Can you work these out from the model? Positions are in its coordinate system, mm. A direction names the side the tool comes from. Coordinates: 2 decimals unless noted, no trailing zeros. Order: outer loops, then holes, each group sorted by start corner. A loop starts at its lowest first (then second) coordinate and runs counter-clockwise, first axis right, second up. Notation, with made-up numbers: (43, 11) - (69, 11) arc R18 ccw to (69, 45) - close; hole circle Ø7 at (34, 83). An arc over 180 degrees is marked (long way). Return JSON: item names as keys, results as strings. Group by question number.
1) For pin 1 Ø3 at (x, z) = (-13.5, -8.5) entering from +Y; pin 2 Ø8.5 at (y, z) = (12.34, -11.91) entering from +X; pin 3 Ø4 at (y, z) = (16.5, -9) entering from -X, each with a flat end and sliding along its axis, tell me the tip position at first contact or that it passes through.
2) Which directions (+Z, -Z, +X, -X, +Y, -Y) give clear straight access to the entire face, cutting with the end or side of a thin tool? Please do faces 1 (the face through (0, 19, -12)), 2 (the face through (-3, 4, -23.81)).
3) Imagine slicing it at B-B (z = -12). Write out the boundary of the cut face in (x, y).
4) Imagine slicing it at A-A (y = 13.5). Write out the boundary of the cut face in (x, z), and give its area (3 significant figures).
5) Imagine slicing it at D-D (y = 16). Write out the boundary of the cut face in (x, z).
6) If we mould it in two halves opening along X, with no side actions, what happens to faces 3 (the face through (-6, 0, -12)), 4 (the face through (-16.026, 2, -12)), 5 (the face through (5, 7, -9))? For each: pulls with the +X half, pulls with the -X half, needs draft (parallel to the pull), parting line crosses it, or undercut.
7) If I drill on line 1 along Y through (x, z) = (-7.75, -14); line 2 along Y through (x, z) = (3, -22.25), over which ranges is the centre line in solid material (lowest first)?
```python
from build123d import *

# Parameters (mm, degrees)
SKETCH2_W           = 16.026033158
SKETCH2_H           = 23.810106406
BOSS_EXTRUDE1_DEPTH = 5
SKETCH3_R           = 5.388558838
BOSS_EXTRUDE2_DEPTH = 5


with BuildPart() as part:
    # Sketch2 → Boss-Extrude1 (new body)
    with BuildSketch(Plane(origin=(0, 0, 0), x_dir=(1, 0, 0), z_dir=(0, 1, 0))):
        with Locations((-8.013016579, 11.905053203)):
            Rectangle(SKETCH2_W, SKETCH2_H)
    extrude(amount=BOSS_EXTRUDE1_DEPTH)

    # Sketch3 → Boss-Extrude2 (add)
    with BuildSketch(Plane(origin=(0, 0, 0), x_dir=(0, 0, -1), z_dir=(1, 0, 0))):
        with BuildLine():
            Line((0, 0), (0, 12.341839421))
            ThreePointArc((0, 12.341839421), (11.905053203, 24.246892624), (23.810106406, 12.341839421))
            Line((23.810106406, 12.341839421), (23.810106406, 0))
            Line((23.810106406, 0), (0, 0))
        make_face()
        with Locations((11.905053203, 12.341839421)):
            Circle(SKETCH3_R, mode=Mode.SUBTRACT)
    extrude(amount=BOSS_EXTRUDE2_DEPTH)


solid = part.part
```
Calculated:
{
 "1": {"pin 1": "y = 5", "pin 2": "through", "pin 3": "x = 0"},
 "2": {"face 1": "+Z, -Z, -X, +Y", "face 2": "-Z, +X, -X, +Y, -Y"},
 "3": {"outline": "(-16.03, 0) - (5, 0) - (5, 6.95) - (0, 6.95) - (0, 5) - (-16.03, 5) - close; (0, 17.73) - (5, 17.73) - (5, 24.25) - (0, 24.25) - close"},
 "4": {"outline": "(0, -23.75) - (5, -23.75) - (5, -17.17) - (0, -17.17) - close; (0, -6.64) - (5, -6.64) - (5, -0.06) - (0, -0.06) - close", "area": "65.9 mm2"},
 "5": {"outline": "(0, -23.23) - (5, -23.23) - (5, -15.86) - (0, -15.86) - close; (0, -7.95) - (5, -7.95) - (5, -0.58) - (0, -0.58) - close"},
 "6": {"face 3": "needs draft", "face 4": "pulls with the -X half", "face 5": "pulls with the +X half"},
 "7": {"line 1": "0 to 5", "line 2": "0 to 18.23"}
}
